from build123d import *

# Parameters (mm, degrees)
SKETCH1_R           = 28
SKETCH1_R_2         = 25
BOSS_EXTRUDE1_DEPTH = 8
BOSS_EXTRUDE2_START = -2
SKETCH1_3_R         = 28
BOSS_EXTRUDE2_DEPTH = 2
SKETCH1_5_R         = 21.6
SKETCH1_5_R_2       = 20.1
BOSS_EXTRUDE3_DEPTH = 5
CUT_EXTRUDE1_START  = -1.9
SKETCH5_R           = 28
CUT_EXTRUDE1_DEPTH  = 1.9
SKETCH10_W          = 2
SKETCH10_H          = 3.423160565
SKETCH10_W_2        = 3.423160565
SKETCH10_H_2        = 2
BOSS_EXTRUDE4_DEPTH = 5


with BuildPart() as part:
    # Sketch1 → Boss-Extrude1 (new body)
    with BuildSketch(Plane(origin=(0, 0, 0), x_dir=(1, 0, 0), z_dir=(0, 1, 0))):
        with Locations(Location((0, 0, 0), (0, 0, 270))):
            Circle(SKETCH1_R)
        with Locations(Location((0, 0, 0), (0, 0, 270))):
            Circle(SKETCH1_R_2, mode=Mode.SUBTRACT)
    extrude(amount=BOSS_EXTRUDE1_DEPTH)

    # Sketch1<3> → Boss-Extrude2 (add)
    with BuildSketch(Plane(origin=(0, 0, 0), x_dir=(1, 0, 0), z_dir=(0, 1, 0)).offset(BOSS_EXTRUDE2_START)):
        with Locations(Location((0, 0, 0), (0, 0, 270))):
            Circle(SKETCH1_3_R)
    extrude(amount=BOSS_EXTRUDE2_DEPTH)

    # Sketch1<5> → Boss-Extrude3 (add)
    with BuildSketch(Plane(origin=(0, 0, 0), x_dir=(1, 0, 0), z_dir=(0, 1, 0))):
        with Locations(Location((0, 0, 0), (0, 0, 270))):
            Circle(SKETCH1_5_R)
        with Locations(Location((0, 0, 0), (0, 0, 270))):
            Circle(SKETCH1_5_R_2, mode=Mode.SUBTRACT)
    extrude(amount=BOSS_EXTRUDE3_DEPTH)

    # Sketch5 → Cut-Extrude1 (cut)
    with BuildSketch(Plane(origin=(0, 8, 0), x_dir=(1, 0, 0), z_dir=(0, 1, 0)).offset(CUT_EXTRUDE1_START)):
        with Locations(Location((0, 0, 0), (0, 0, 270))):
            Circle(SKETCH5_R)
    extrude(amount=CUT_EXTRUDE1_DEPTH, mode=Mode.SUBTRACT)

    # Sketch10 → Boss-Extrude4 (add)
    with BuildSketch(Plane(origin=(0, 0, 0), x_dir=(1, 0, 0), z_dir=(0, 1, 0))):
        with Locations((0, -23.288419717)):
            Rectangle(SKETCH10_W, SKETCH10_H)
        with Locations((-23.288419717, 0)):
            Rectangle(SKETCH10_W_2, SKETCH10_H_2)
        with Locations((23.288419717, 0)):
            Rectangle(SKETCH10_W_2, SKETCH10_H_2)
        with Locations((0, 23.288419717)):
            Rectangle(SKETCH10_W, SKETCH10_H)
    extrude(amount=BOSS_EXTRUDE4_DEPTH)


solid = part.part
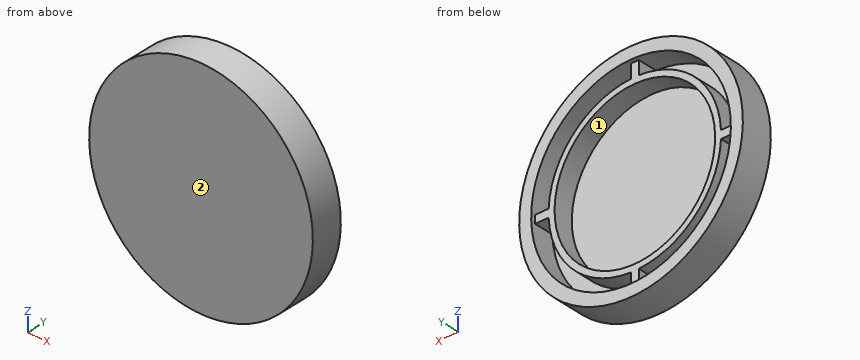
Can you work these out from the model? Positions are in its coordinate system, mm. Face numbers are marked on the shaded views. A direction names the side the tool comes from. Give positions to 0.01 mm unless a question says otherwise; leave off trailing zeros. Order: outer loops, then holes, each group sorted by start corner. A loop starts at its lowest first (then second) coordinate and runs counter-clockwise, first axis right, second up. Notation, with made-up numbers: M 84,75 L 123,75 A29 ccw 123,108 Z; hole C 42,53.5 d5. An arc over 180 degrees is marked long. Use one line per item in the form item = value.
Item 1: Will these pins go through, and if not, where does the flat tip stop? pin 1 Ø19 at (x, z) = (7.5, -13) entering from +Y; pin 2 Ø1 at (x, z) = (17.5, 0.5) entering from +Y; pin 3 Ø3 at (y, z) = (5, 15) entering from -X.
Values follow:
pin_1 = 5
pin_2 = 0
pin_3 = -24.53
Item 2: If we section it at D-D, the plane x = 12: Write out the boundary of the cut face in (y, z), and give its area (3 significant figures).
Values follow:
outline = M -2,-25.3 L 6.1,-25.3 L 6.1,-21.93 L 0,-21.93 L 0,-17.96 L 5,-17.96 L 5,-16.12 L 0,-16.12 L 0,16.12 L 5,16.12 L 5,17.96 L 0,17.96 L 0,21.93 L 6.1,21.93 L 6.1,25.3 L -2,25.3 Z
area = 161 mm^2
Item 3: For the marked faces 1 and 2, which set-ups out of +Z, -Z, +X, -X, +Y, -Y let a thin tool reach every point of the face, with its end or its side?
Values follow:
face_1 = +Y
face_2 = +Z, -Z, +X, -X, -Y
Item 4: If we section it at B-B, the plane x = 0: Write out the boundary of the cut face in (y, z).
Values follow:
outline = M -2,-28 L 6.1,-28 L 6.1,-25 L 5,-25 L 5,-20.1 L 0,-20.1 L 0,20.1 L 5,20.1 L 5,25 L 6.1,25 L 6.1,28 L -2,28 Z
Item 5: If we section it at A-A, the plane y = 3: Write out the boundary of the cut face in (x, z), and give its area (3 significant figures).
Values follow:
outline = C 0,0 d56; hole M -24.98,-1 A25 ccw -1,-24.98 L -1,-21.58 A21.6 cw -21.58,-1 Z; hole M -24.98,1 L -21.58,1 A21.6 cw -1,21.58 L -1,24.98 A25 ccw Z; hole C 0,0 d40.2; hole M 1,-24.98 A25 ccw 24.98,-1 L 21.58,-1 A21.6 cw 1,-21.58 Z; hole M 1,21.58 A21.6 cw 21.58,1 L 24.98,1 A25 ccw 1,24.98 Z
area = 723 mm^2
Item 6: If we section it at C-C, the plane z = 0: Write out the boundary of the cut face in (x, y), and give its area (3 significant figures).
Values follow:
outline = M -28,-2 L 28,-2 L 28,6.1 L 25,6.1 L 25,5 L 20.1,5 L 20.1,0 L -20.1,0 L -20.1,5 L -25,5 L -25,6.1 L -28,6.1 Z
area = 198 mm^2
Item 7: If I drill on line 1 along X through (y, z) = (1.4, 0); line 2 along Z through (x, y) = (18, 2.75); line 3 along Z through (x, y) = (-3.5, 4), over which ranges is the centre line in solid material (lowest first)? Write a range as [from, to].
Values follow:
line_1 = [-28, -20.1], [20.1, 28]
line_2 = [-21.45, -17.35], [-11.94, -8.94], [8.94, 11.94], [17.35, 21.45]
line_3 = [-27.78, -24.75], [-21.31, -19.79], [19.79, 21.31], [24.75, 27.78]
